Geometry: see drawing. Coordinates: mm, zero at the bounding-box minimum. A direction names the side the tool comes from. Coordinates: 2 decimals unless noted, no trailing zeros. Use one line per item in the form item = value.
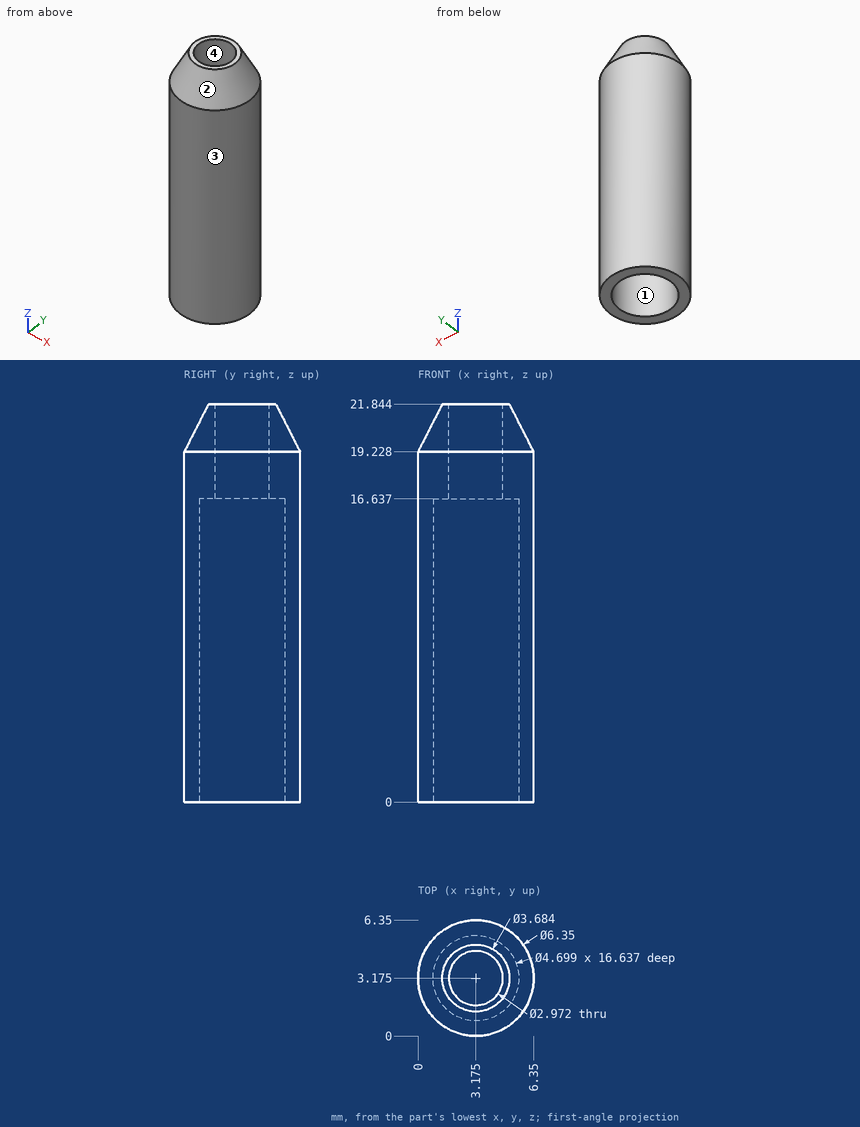
1) Material intervals for probe 1 along X at (y, z) = (3.25, 11.5); probe 2 along Z at (x, y) = (2.25, 4.5); probe 3 along Y at (x, z) = (3.25, 19), sorted ascending. Write a range as from..to.
Results found:
probe_1 = 0..0.83, 5.52..6.35
probe_2 = 16.64..21.84
probe_3 = 0..1.69, 4.66..6.35
2) Contact query for a flat-ended pin moving along its axis: P1, Ø1, axis at y = 4, z = 10, coming from the -X side. Output: stop coordinate, or through.
Results found:
P1 = 0.02
3) Pull-direction query (Y, two-part tool) for the marked faces 3 and 4; classes: released by +Y, released by -Y, zero draft, split by the parting line, or undercut.
Results found:
face_3 = split by the parting line
face_4 = undercut
4) Access query for the marked faces 1 and 2. Directions: +Z, -Z, +X, -X, +Y, -Y. A direction counts if a zero-diameter tool reaches every point of the face in a straight line with its end or side. Return the directions, or none.
Results found:
face_1 = -Z
face_2 = +Z
